Here's how the part is built. I have some questions about the finished solid (model axes, mm). A direction names the side the tool comes from. Coordinates: 2 decimals unless noted, no trailing zeros. Write each loop counter-clockwise with the first axis right and the second up, starting at its lowest first coordinate (ties: lowest second). Pieces come first, ordered by that corner, then holes. Notation, with made-up numbers: (-19.75, 20) -> (-10.75, 20) arc R11 ccw to (-10.75, 30) -> close; hole circle Ø1 at (2.25, 85.25). An arc over 180 degrees is marked (long way). Use CSV: the item, a comma, the result in double quotes. Start each with the question number.
```python
from build123d import *

# Parameters (mm, degrees)
SKETCH1_R           = 3
BOSS_EXTRUDE1_DEPTH = 23
CHAMFER1_SIZE       = 0.5
CUT_EXTRUDE1_DEPTH  = 6


with BuildPart() as part:
    # Sketch1 → Boss-Extrude1 (new body, symmetric)
    with BuildSketch(Plane(origin=(0, 0, 0), x_dir=(0, 0, -1), z_dir=(1, 0, 0))):
        Circle(SKETCH1_R)
    extrude(amount=BOSS_EXTRUDE1_DEPTH, both=True)

    # Chamfer1
    chamfer1_edges = [part.edges().sort_by_distance(p)[0] for p in [
        (-23, 0, 3),
        (23, 0, 3),
    ]]
    chamfer(chamfer1_edges, length=CHAMFER1_SIZE)

    # Sketch2 → Cut-Extrude1 (cut)
    with BuildSketch(Plane(origin=(23, 0, 0), x_dir=(0, 0, -1), z_dir=(1, 0, 0))):
        with BuildLine():
            Line((-2.236067977, 2), (2.236067977, 2))
            ThreePointArc((2.236067977, 2), (0, 3), (-2.236067977, 2))
        make_face()
    cut_extrude1 = extrude(amount=-CUT_EXTRUDE1_DEPTH, mode=Mode.SUBTRACT)

    # Mirror1: Cut-Extrude1 across plane
    add(cut_extrude1.mirror(Plane(origin=(0, 0, 0), x_dir=(0, 0, 1), z_dir=(1, 0, 0))), mode=Mode.SUBTRACT)


solid = part.part
```
Item 1: I want a section at B-B on x = -7. Please give me the cut outline in (y, z).
Item 2: Which directions (+Z, -Z, +X, -X, +Y, -Y) give clear straight access to the entire face, cutting with the end or side of a thin tool? Please do faces 1 (the flat face through (-20, 2, 0)), 2 (the conical face through (22.865, -2.634, 0.092)), 3 (the flat face through (17, 2.4, 0)).
Item 3: I want a section at C-C on x = 19. Please give me the cut outline in (y, z), then the cut area to 3 significant figures.
Item 4: I want a section at A-A on z = 0. Please give me the cut outline in (x, y), then the cut area to 3 significant figures.
Item 5: I'm going to push flat-ended pins straight in: pin 1 (0.5 mm diameter, centred on y = 2.5, z = 0, fed in from +X); pin 2 (2 mm diameter, centred on x = -19.5, z = 1, fed in from +Y). Where does each tip first touch, or does it pass through?
Item 6: If I drill on line 1 along Y through (x, z) = (7.5, -0.15); line 2 along Z through (x, y) = (-19, 1.8); line 3 along Z through (x, y) = (6, -0.85), over which ranges is the centre line in solid material (lowest first)?
Geometry says:
1,outline,"circle Ø6 at (0, 0)"
2,face 1,"+Z, -Z, -X, +Y"
2,face 2,"+X"
2,face 3,"+Z, -Z, +X, +Y"
3,outline,"(2, -2.24) -> (2, 2.24) arc R3 ccw (long way) to start"
3,area,"25.2 mm2"
4,outline,"(-23, -2.5) -> (-22.5, -3) -> (22.5, -3) -> (23, -2.5) -> (23, 2) -> (17, 2) -> (17, 3) -> (-17, 3) -> (-17, 2) -> (-23, 2) -> close"
4,area,"264 mm2"
5,pin 1,"x = 17"
5,pin 2,"y = 2"
6,line 1,"-3 to 3"
6,line 2,"-2.4 to 2.4"
6,line 3,"-2.88 to 2.88"
